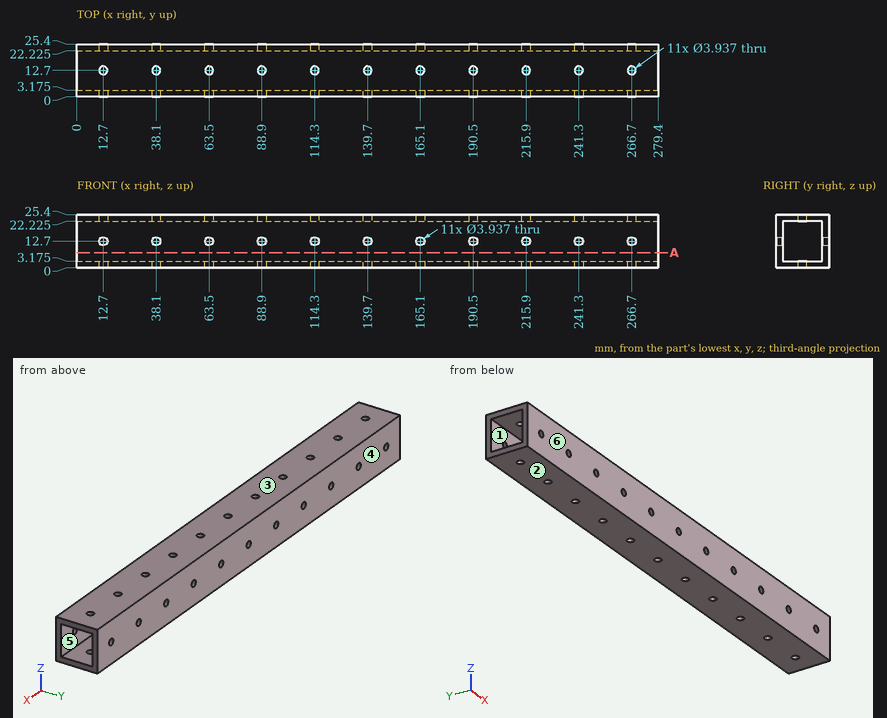
Design review of the part shown in the three views and the two pictorial views. Dimensions are in mm from the part's minimum x, y and z. A direction names the side the tool comes from. Coordinates: 2 decimals unless noted, no trailing zeros. Order: outer loops, then holes, each group sorted by start corner. A loop starts at its lowest first (then second) coordinate and runs counter-clockwise, first axis right, second up.
Item 1: Take a section at A-A, the plane z = 7.25. Write out the cut boundary in (x, y) (3 decimals).
Item 2: For line 1 (Z direction, x = 165.5, y = 15.5) (3 decimals); line 2 (Z direction, x = 88.9, y = 23.5), list the stretches that pass through material, from the lowest coordinate up.
Item 3: For the marked faces 5 and 6, list the 3-axis set-ups (+Z, -Z, +X, -X, +Y, -Y) from which the entire face can be reached by the end or side of a thin tool; tool diameter is ignored.
Item 4: The part is to be moulded in two halves that separate along Z. For the marked faces 1, 2, 3 and 4, say which applies: pulls with the +Z half, pulls with the -Z half, needs draft (parallel to the pull), parting line crosses it, or undercut.
Item 5: For pin 1 Ø3.5 at (x, y) = (139.7, 12.7) entering from +Z, flat-tipped, find the tip position at first contact; note if it passes through.
The answers:
1. outline: (0, 0) - (279.4, 0) - (279.4, 3.175) - (0, 3.175) - close; (0, 22.225) - (279.4, 22.225) - (279.4, 25.4) - (0, 25.4) - close
2. line 1: z = 0 to 3.175, 22.225 to 25.4
2. line 2: z = 0 to 10.73, 14.67 to 25.4
3. face 5: +X, -X
3. face 6: +Z, -Z, +X, -X, -Y
4. face 1: undercut
4. face 2: pulls with the -Z half
4. face 3: pulls with the +Z half
4. face 4: needs draft
5. pin 1: passes through
